from build123d import *

# Parameters (mm, degrees)
SKETCH_1_W               = 42
SKETCH_1_H               = 42
EXTRUDE_1_DEPTH          = 33
CHAMFER_1_SIZE           = 5
EXTRUDE_2_DEPTH          = 12
EXTRUDE_START            = -10
EXTRUDE_3_DEPTH          = 35
SKETCH_5_W               = 22
SKETCH_5_H               = 36
EXTRUDE_4_DEPTH          = 1.5
EXTRUDE_5_DEPTH          = 22
PATTERN_CIRCULAR_1_COUNT = 3
CUT_EXTRUDE_1_DEPTH      = 65.991772006
CUT_EXTRUDE_2_DEPTH      = 59.741772006
CUT_EXTRUDE_3_DEPTH      = 65.991772006


with BuildPart() as part:
    # Sketch 1 → Extrude 1 (new body)
    with BuildSketch(Plane(origin=(0, 0, 0), x_dir=(1, 0, 0), z_dir=(0, 1, 0))):
        Rectangle(SKETCH_1_W, SKETCH_1_H)
    extrude(amount=EXTRUDE_1_DEPTH)

    # Chamfer 1
    chamfer_1_edges = [part.edges().sort_by_distance(p)[0] for p in [
        (21, 16.5, 21),
        (-21, 16.5, 21),
        (-21, 16.5, -21),
        (21, 16.5, -21),
    ]]
    chamfer(chamfer_1_edges, length=CHAMFER_1_SIZE)

    # Sketch 3 → Extrude 2 (add)
    with BuildSketch(Plane(origin=(0, 0, 0), x_dir=(1, 0, 0), z_dir=(0, 1, 0))):
        with BuildLine():
            Line((-11, 27.910571474), (-11, 42))
            Line((-11, 42), (11, 42))
            Line((11, 42), (11, 27.910571474))
            ThreePointArc((11, 27.910571474), (25.980762114, 15), (29.671263931, -4.429006295))
            Line((29.671263931, -4.429006295), (41.873066959, -11.473720558))
            Line((41.873066959, -11.473720558), (30.873066959, -30.526279442))
            Line((30.873066959, -30.526279442), (18.671263931, -23.481565179))
            ThreePointArc((18.671263931, -23.481565179), (0, -30), (-18.671263931, -23.481565179))
            Line((-18.671263931, -23.481565179), (-30.873066959, -30.526279442))
            Line((-30.873066959, -30.526279442), (-41.873066959, -11.473720558))
            Line((-41.873066959, -11.473720558), (-29.671263931, -4.429006295))
            ThreePointArc((-29.671263931, -4.429006295), (-25.980762114, 15), (-11, 27.910571474))
        make_face()
    extrude(amount=-EXTRUDE_2_DEPTH)

    # Sketch 4 → Extrude 3 (add)
    with BuildSketch(Plane(origin=(0, -12, 0), x_dir=(-1, 0, 0), z_dir=(0, -1, 0)).offset(EXTRUDE_START)):
        Polygon((-11, 30), (-11, 46.410571474), (11, 46.410571474), (11, 30), (12.5, 30), (12.5, 47.910571474), (-12.5, 47.910571474), (-12.5, 30), align=None)
    extrude_3 = extrude(amount=EXTRUDE_3_DEPTH)

    # Sketch 5 → Extrude 4 (add)
    with BuildSketch(Plane(origin=(0, -37, 0), x_dir=(-1, 0, 0), z_dir=(0, -1, 0))):
        with Locations((0, 28.410571474)):
            Rectangle(SKETCH_5_W, SKETCH_5_H)
    extrude_4 = extrude(amount=-EXTRUDE_4_DEPTH)

    # Sketch 6 → Extrude 5 (add)
    with BuildSketch(Plane(origin=(11, 0, 0), x_dir=(0, 0, -1), z_dir=(1, 0, 0))):
        Polygon((10.410571474, -37), (47.910571474, -37), (29.160571474, -137), align=None)
    extrude_5 = extrude(amount=-EXTRUDE_5_DEPTH)

    # Pattern Circular 1: Extrude 3, Extrude 4, Extrude 5 ×3 about axis
    pattern_circular_1_axis = Axis((0, 0, 0), (0, 1, 0))
    for i in range(1, PATTERN_CIRCULAR_1_COUNT):
        add(extrude_3.rotate(pattern_circular_1_axis, i * 360 / PATTERN_CIRCULAR_1_COUNT))
        add(extrude_4.rotate(pattern_circular_1_axis, i * 360 / PATTERN_CIRCULAR_1_COUNT))
        add(extrude_5.rotate(pattern_circular_1_axis, i * 360 / PATTERN_CIRCULAR_1_COUNT))

    # Sketch 7 → Cut-Extrude 1 (cut, through all)
    with BuildSketch(Plane(origin=(5.5, 0, -9.526279442), x_dir=(-0.866025404, 0, -0.5), z_dir=(0.5, 0, -0.866025404))):
        Polygon((-40.245205142, -56), (-17.739434055, -56), (-14.926151928, -41), (-26.07846167, -41), (-43.090866325, -41), align=None)
        Polygon((-39.48636216, -60), (-18.489642622, -60), (-21.302924749, -75), (-36.640700976, -75), align=None)
        Polygon((-35.881857994, -79), (-22.053133316, -79), (-24.866415443, -94), (-33.036196811, -94), align=None)
        Polygon((-28.927933406, -115.655406991), (-25.61662401, -98), (-32.277353829, -98), align=None)
    extrude(amount=-CUT_EXTRUDE_1_DEPTH, mode=Mode.SUBTRACT)

    # Sketch 8 → Cut-Extrude 2 (cut, through all)
    with BuildSketch(Plane(origin=(11, 0, 0), x_dir=(0, 0, -1), z_dir=(1, 0, 0))):
        Polygon((17.91967612, -57.599451379), (40.425447207, -57.599451379), (43.238729334, -42.599451379), (32.086419592, -42.599451379), (15.074014936, -42.599451379), align=None)
        Polygon((18.678519102, -61.599451379), (39.675238639, -61.599451379), (36.861956513, -76.599451379), (21.524180285, -76.599451379), align=None)
        Polygon((22.283023267, -80.599451379), (36.111747945, -80.599451379), (33.298465818, -95.599451379), (25.12868445, -95.599451379), align=None)
        Polygon((29.236947856, -117.25485837), (32.548257251, -99.599451379), (25.887527433, -99.599451379), align=None)
    extrude(amount=-CUT_EXTRUDE_2_DEPTH, mode=Mode.SUBTRACT)

    # Sketch 9 → Cut-Extrude 3 (cut, through all)
    with BuildSketch(Plane(origin=(-5.5, 0, -9.526279442), x_dir=(-0.866025404, 0, 0.5), z_dir=(-0.5, 0, -0.866025404))):
        Polygon((18.364266378, -57.83156369), (40.870037466, -57.83156369), (43.683319592, -42.83156369), (32.531009851, -42.83156369), (15.518605195, -42.83156369), align=None)
        Polygon((19.123109361, -61.83156369), (40.119828898, -61.83156369), (37.306546771, -76.83156369), (21.968770544, -76.83156369), align=None)
        Polygon((22.727613526, -80.83156369), (36.556338204, -80.83156369), (33.743056077, -95.83156369), (25.573274709, -95.83156369), align=None)
        Polygon((29.681538115, -117.486970681), (32.99284751, -99.83156369), (26.332117691, -99.83156369), align=None)
    extrude(amount=-CUT_EXTRUDE_3_DEPTH, mode=Mode.SUBTRACT)


solid = part.part
Check sheet for the modelled part. Datum: model origin and axes. Units: mm. A direction names the side the tool comes from. Round coordinates to 2 decimals unless told otherwise and drop trailing zeros. Order: outer loops, then holes, each group sorted by start corner. A loop starts at its lowest first (then second) coordinate and runs counter-clockwise, first axis right, second up.
(1) Go/stop test with flat-tipped pins: P1, Ø14, axis at x = 35.5, z = 13, coming from the +Y side; P2, Ø17.5, axis at x = -2, y = -18.5, coming from the +Z side; P3, Ø10, axis at y = -10.5, z = -38, coming from the +X side. Record where each tip stops, or that it passes through.
(2) Cross-section at A-A, the plane y = -28.5. Enter the section's corners in (x, z).
(3) Access from +Z, -Z, +X, -X, +Y, -Y to the whole of each face (thin tool, end or side, straight path). Record for faces 4 (the flat face through (-21, 16, 0)), 5 (the flat face through (27.595, -19.255, 30.366)), 6 (the flat face through (-36.3, -5.92, 21.13)).
(4) Scan lines: probe 1 along X at (y, z) = (-33, -38); probe 2 along X at (y, z) = (-88, 19); probe 3 along X at (y, z) = (-56.5, 17). Record each from-to range of solid material in increasing order.
(5) Cross-section at C-C, the plane y = -104. Enter the section's corners in (x, z), and give its area (3 significant figures).
(6) Cross-section at B-B, the plane z = -13. Enter the section's corners in (x, y), and give its area (3 significant figures).
(7) Cross-section at D-D, the plane y = 8. Enter the section's corners in (x, z).
(8) Draft check along Y on faces 1 (the flat face through (0, -61.599, -29)), 2 (the flat face through (0.154, -87.7, -19.917)), 3 (the flat face through (0, -6, -42)). Enter one of: pulls with the +Y half, pulls with the -Y half, needs draft (parallel to the pull), parting line crosses it, or undercut.
Check sheet entries:
1. P1: stops at y = 0
1. P2: stops at z = 30
1. P3: stops at x = 12.5
2. outline: (-47.74, 13.13) - (-32.23, 4.17) - (-31.48, 5.47) - (-45.69, 13.68) - (-34.69, 32.73) - (-20.48, 24.53) - (-19.73, 25.83) - (-35.24, 34.78) - close; (-12.5, -47.91) - (12.5, -47.91) - (12.5, -30) - (11, -30) - (11, -46.41) - (-11, -46.41) - (-11, -30) - (-12.5, -30) - close; (19.73, 25.83) - (20.48, 24.53) - (34.69, 32.73) - (45.69, 13.68) - (31.48, 5.47) - (32.23, 4.17) - (47.74, 13.13) - (35.24, 34.78) - close
3. face 4: +Z, -Z, -X, +Y
3. face 5: +Z, +Y, -Y
3. face 6: +Y
4. probe 1: x = -12.5 to -11, 11 to 12.5
4. probe 2: x = -33.31 to -29.69, -16.84 to -12.09, 12.09 to 16.44, 28.49 to 33.31
4. probe 3: x = -41.29 to -37.67, -11.1 to -7.44, 7.44 to 41.29
5. outline: (-36.11, 8.15) - (-33.4, 6.58) - (-22.4, 25.63) - (-25.11, 27.2) - close; (-28.99, 4.04) - (-25.4, 1.96) - (-14.4, 21.01) - (-17.99, 23.09) - close; (-11, -35.35) - (11, -35.35) - (11, -31.72) - (-11, -31.72) - close; (-11, -26.72) - (11, -26.72) - (11, -22.97) - (-11, -22.97) - close; (14.4, 21.01) - (25.4, 1.96) - (28.66, 3.84) - (17.66, 22.9) - close; (21.47, 25.1) - (32.47, 6.04) - (36.11, 8.15) - (25.11, 27.2) - close
5. area: 498 mm2
6. outline: (-27.04, -12) - (27.04, -12) - (27.04, 0) - (21, 0) - (21, 33) - (-21, 33) - (-21, 0) - (-27.04, 0) - close; (-11, -50.81) - (11, -50.81) - (11, -35.5) - (-11, -35.5) - close
6. area: 2,370 mm2
7. outline: (-21, -16) - (-16, -21) - (16, -21) - (21, -16) - (21, 16) - (16, 21) - (-16, 21) - (-21, 16) - close
8. face 1: undercut
8. face 2: pulls with the -Y half
8. face 3: needs draft
